Input: dimensioned drawing with shaded views. Units: mm. Origin: part minimum x, y, z. Coordinates: 2 decimals unless noted, no trailing zeros. Order: outer loops, then holes, each group sorted by start corner. A loop starts at its lowest first (then second) coordinate and runs counter-clockwise, first axis right, second up. Notation, with made-up numbers: (-22, 57.5) -> (-9, 57.5) arc R22 ccw to (-9, 76.5) -> close; hole circle Ø3 at (-1.75, -10). An arc over 180 degrees is marked (long way). Answer as CSV lines item,"result".
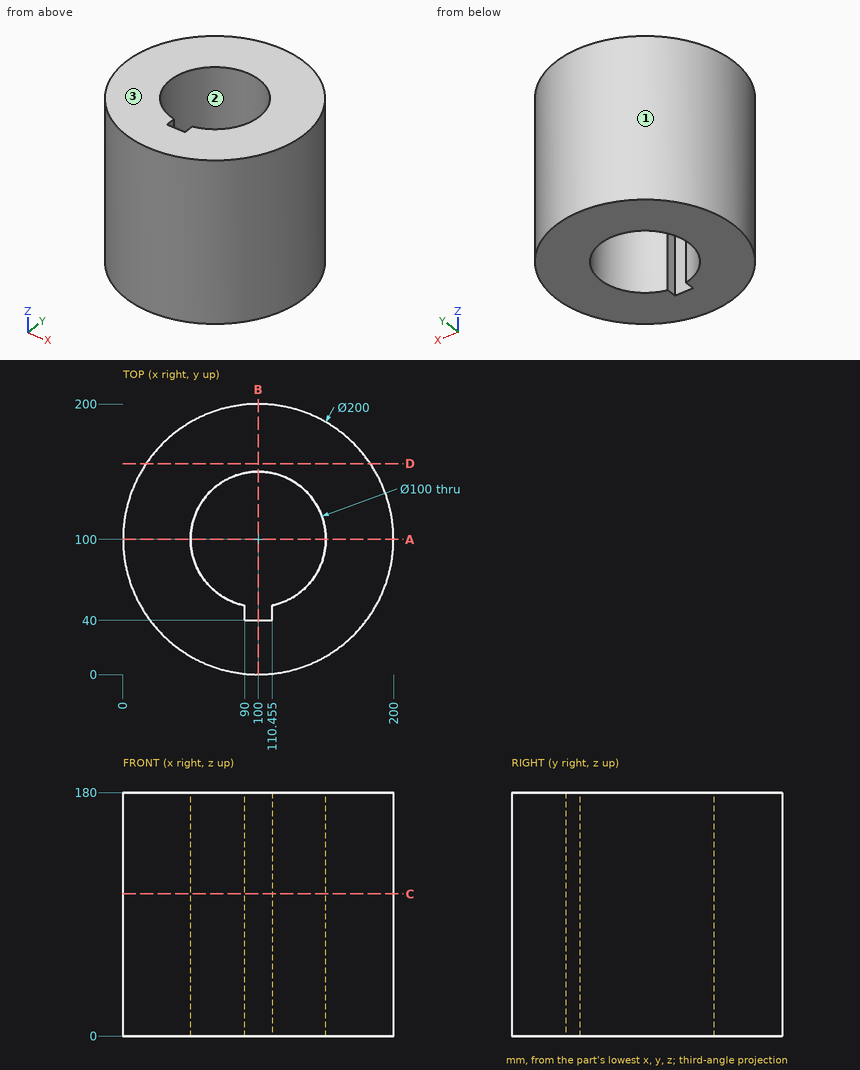
1. Mould query, pull axis Y, two halves, no side actions, for the marked faces 1, 2 and 3. Classes: released by +Y, released by -Y, zero draft, split by the parting line, or undercut.
Findings:
face 1,"split by the parting line"
face 2,"undercut"
face 3,"zero draft"
2. Ray query, line 1 along Y through (x, z) = (100, 88.5); line 2 along X through (y, z) = (59, 14) (1 decimal); line 3 along Y through (x, z) = (125, 8) (1 decimal). Return the intervals inside material, ascending.
Findings:
line 1,"y = 0 to 40, 150 to 200"
line 2,"x = 8.8 to 71.4, 128.6 to 191.2"
line 3,"y = 3.2 to 56.7, 143.3 to 196.8"
3. Cut plane A-A (y = 100). Return the cut outline in (x, z), plus the area to 3 significant figures.
Findings:
outline,"(0, 0) -> (50, 0) -> (50, 180) -> (0, 180) -> close; (150, 0) -> (200, 0) -> (200, 180) -> (150, 180) -> close"
area,"18,000 mm2"
4. Cut plane D-D (y = 156). Return the cut outline in (x, z).
Findings:
outline,"(17.15, 0) -> (182.85, 0) -> (182.85, 180) -> (17.15, 180) -> close"
5. Cut plane B-B (x = 100). Return the cut outline in (y, z).
Findings:
outline,"(0, 0) -> (40, 0) -> (40, 180) -> (0, 180) -> close; (150, 0) -> (200, 0) -> (200, 180) -> (150, 180) -> close"
6. Contact query for flat-ended pins moving along their axis: pin 1 (1 mm diameter, centred on y = 65.5, z = 94, fed in from -X); pin 2 (1 mm diameter, centred on x = 124.5, z = 150, fed in from +Y); pin 3 (8 mm diameter, centred on y = 73, z = 97, fed in from -X). Output: stop coordinate, or through.
Findings:
pin 1,"stops at x = 5.96"
pin 2,"stops at y = 197.08"
pin 3,"stops at x = 2.68"
7. Cut plane C-C (z = 105). Return the cut outline in (x, y) (1 decimal), plus the area to 4 significant figures.
Findings:
outline,"circle Ø200 at (100, 100); hole (90, 40) -> (110.5, 40) -> (110.5, 51.1) arc R50 ccw (long way) to (90, 51) -> close"
area,"23,350 mm2"
